```python
from build123d import *

# Parameters (mm, degrees)
BOSS_EXTRUDE1_DEPTH = 5
SKETCH2_W           = 50.6
SKETCH2_H           = 22.6
SKETCH2_W_2         = 48
SKETCH2_H_2         = 20
BOSS_EXTRUDE2_DEPTH = 7.9
SKETCH3_R           = 1.1
CUT_EXTRUDE1_DEPTH  = 3
BOSS_EXTRUDE3_DEPTH = 3
CHAMFER1_SIZE       = 1
SKETCH5_R           = 3.1
CUT_EXTRUDE2_DEPTH  = 3


with BuildPart() as part:
    # Sketch1 → Boss-Extrude1 (new body)
    with BuildSketch(Plane.XY):
        Polygon((24, 12.55), (6.08, 12.55), (-6.08, 12.55), (-24, 12.55), (-24, -7.45), (24, -7.45), align=None)
    extrude(amount=BOSS_EXTRUDE1_DEPTH)

    # Sketch2 → Boss-Extrude2 (add)
    with BuildSketch(Plane.XY.offset(5)):
        with Locations((0, 2.55)):
            Rectangle(SKETCH2_W, SKETCH2_H)
        with Locations((0, 2.55)):
            Rectangle(SKETCH2_W_2, SKETCH2_H_2, mode=Mode.SUBTRACT)
    extrude(amount=-BOSS_EXTRUDE2_DEPTH)

    # Sketch3 → Cut-Extrude1 (cut)
    with BuildSketch(Plane(origin=(0, 0, 0), x_dir=(-1, 0, 0), z_dir=(0, 0, -1))):
        with Locations((-18.5, 0)):
            Circle(SKETCH3_R)
        with Locations((18.5, 0)):
            Circle(SKETCH3_R)
    extrude(amount=-CUT_EXTRUDE1_DEPTH, mode=Mode.SUBTRACT)

    # Sketch4 → Boss-Extrude3 (add)
    with BuildSketch(Plane.XY.offset(5)):
        with BuildLine():
            Line((25.3, -7.439559179), (31.3, -7.439559179))
            ThreePointArc((31.3, -7.439559179), (38.729997149, -0.00956203), (31.3, 7.42043512))
            Line((31.3, 7.42043512), (25.3, 7.42043512))
            Line((25.3, 7.42043512), (25.3, -7.439559179))
        make_face()
        with BuildLine():
            Line((-25.3, -7.439559179), (-31.3, -7.439559179))
            ThreePointArc((-31.3, -7.439559179), (-38.729997149, -0.00956203), (-31.3, 7.42043512))
            Line((-31.3, 7.42043512), (-25.3, 7.42043512))
            Line((-25.3, 7.42043512), (-25.3, -7.439559179))
        make_face()
    extrude(amount=-BOSS_EXTRUDE3_DEPTH)

    # Chamfer1
    chamfer1_edges = [part.edges().sort_by_distance(p)[0] for p in [
        (25.3, -0.00956203, 2),
        (25.3, -7.439559179, 3.5),
        (25.3, 7.42043512, 3.5),
        (-25.3, -0.00956203, 2),
        (-25.3, 7.42043512, 3.5),
        (-25.3, -7.439559179, 3.5),
    ]]
    chamfer(chamfer1_edges, length=CHAMFER1_SIZE)

    # Sketch5 → Cut-Extrude2 (cut)
    with BuildSketch(Plane(origin=(0, 0, 2), x_dir=(-1, 0, 0), z_dir=(0, 0, -1))):
        with Locations((-33.1, -0.00956203)):
            Circle(SKETCH5_R)
        with Locations((33.1, -0.00956203)):
            Circle(SKETCH5_R)
    extrude(amount=-CUT_EXTRUDE2_DEPTH, mode=Mode.SUBTRACT)


solid = part.part
```
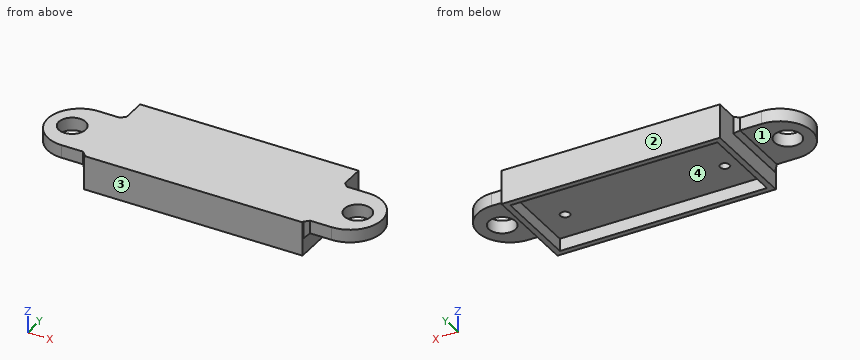
Input: part model. Units: mm. Frame: model coordinates. Face numbers are marked on the shaded views. A direction names the side the tool comes from. Give positions to 0.01 mm unless a question says otherwise; leave off trailing zeros. Loops run counter-clockwise (first coordinate to the right, second up) from the corner with the lowest first, then second, coordinate; pieces in that order, holes last. Notation, with made-up numbers: M 39.5,53 L 67.5,53 A22 cw 67.5,88 Z; hole C 27,39 d10. An arc over 180 degrees is marked long. Answer as CSV lines item,"result". Start each with the question number.
1. Reachability of the marked faces 1 and 2 from +Z, -Z, +X, -X, +Y, -Y: full face, straight path, thin tool, end or side. Return the list, or none.
2. Section D-D on y = 5.5. Return loops of the section in (x, z), plus the area to 3 significant figures.
3. Section A-A on z = -1. Return loops of the section in (x, y).
4. Pin query (flat end, axial travel): P1, Ø13.5, axis at x = 33, y = -2, coming from the -Z side; P2, Ø4, axis at x = -3, y = -0.5, coming from the -Z side; P3, Ø1.5, axis at y = 9.5, z = 2.5, coming from the -X side. Return the tip coordinate at first contact, or that it passes through.
5. Section B-B on y = 11. Return loops of the section in (x, z), plus the area to 3 significant figures.
6. Line query: L1, parallel to X at y = -1, z = -2; L2, parallel to Y at x = 5, z = -1; L3, parallel to Y at x = 18.5, z = 1.2. Output: solid intervals per line, ascending.
7. Section C-C on x = -18.5. Return loops of the section in (y, z), plus the area to 3 significant figures.
8. Pull-direction query (X, two-part tool) for the marked faces 3 and 4; classes: released by +X, released by -X, zero draft, split by the parting line, or undercut.
Computed values:
1,face 1,"-Z, -X, +Y, -Y"
1,face 2,"+Z, -Z, +X, -X, +Y"
2,outline,"M -36.28,2 L -26.3,2 L -25.3,1 L -25.3,-2.9 L -24,-2.9 L -24,0 L 24,0 L 24,-2.9 L 25.3,-2.9 L 25.3,1 L 26.3,2 L 36.28,2 L 36.28,5 L -36.28,5 Z"
2,area,"327 mm²"
3,outline,"M -25.3,-8.75 L 25.3,-8.75 L 25.3,13.85 L -25.3,13.85 Z; hole M -24,-7.45 L 24,-7.45 L 24,12.55 L -24,12.55 Z"
4,P1,"stops at z = 1.95"
4,P2,"stops at z = 0"
4,P3,"stops at x = -25.3"
5,outline,"M -25.3,-2.9 L -24,-2.9 L -24,0 L 24,0 L 24,-2.9 L 25.3,-2.9 L 25.3,5 L -25.3,5 Z"
5,area,"261 mm²"
6,L1,"x = -25.3 to -24, 24 to 25.3"
6,L2,"y = -8.75 to -7.45, 12.55 to 13.85"
6,L3,"y = -8.75 to -1.1, 1.1 to 13.85"
7,outline,"M -8.75,-2.9 L -7.45,-2.9 L -7.45,0 L -1.1,0 L -1.1,3 L 1.1,3 L 1.1,0 L 12.55,0 L 12.55,-2.9 L 13.85,-2.9 L 13.85,5 L -8.75,5 Z"
7,area,"114 mm²"
8,face 3,"zero draft"
8,face 4,"undercut"
